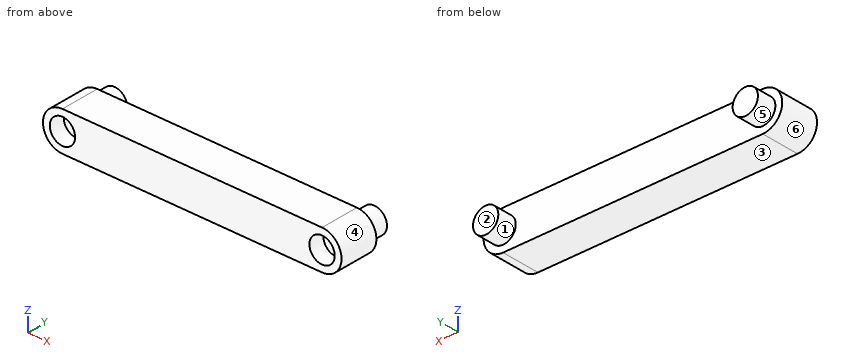
from build123d import *

# Parameters (mm, degrees)
BOSS_EXTRUDE1_DEPTH = 15
SKETCH2_R           = 9.75
CUT_EXTRUDE1_DEPTH  = 117.940155635
BOSS_EXTRUDE2_START = 30
SKETCH2_2_R         = 9.75
BOSS_EXTRUDE2_DEPTH = 30
SKETCH2_3_R         = 9.75
BOSS_EXTRUDE3_DEPTH = 3


with BuildPart() as part:
    # Sketch1 → Boss-Extrude1 (new, symmetric)
    with BuildSketch(Plane(origin=(0, 0, 0), x_dir=(1, 0, 0), z_dir=(0, 1, 0))):
        with BuildLine():
            Line((-100, 15), (100, 15))
            ThreePointArc((100, 15), (115, 0), (100, -15))
            Line((100, -15), (-100, -15))
            ThreePointArc((-100, -15), (-115, 0), (-100, 15))
        make_face()
    extrude(amount=BOSS_EXTRUDE1_DEPTH, both=True)

    # Sketch2 → Cut-Extrude1 (cut, through all)
    with BuildSketch(Plane(origin=(0, 0, 0), x_dir=(1, 0, 0), z_dir=(0, 1, 0))):
        with Locations(Location((100, 0, 0), (0, 0, 270))):
            Circle(SKETCH2_R)
        with Locations(Location((-100, 0, 0), (0, 0, 270))):
            Circle(SKETCH2_R)
    extrude(amount=-CUT_EXTRUDE1_DEPTH, mode=Mode.SUBTRACT)

    # Sketch2_2 → Boss-Extrude2 (add)
    with BuildSketch(Plane(origin=(0, 0, 0), x_dir=(1, 0, 0), z_dir=(0, 1, 0)).offset(BOSS_EXTRUDE2_START)):
        with Locations(Location((100, 0, 0), (0, 0, 270))):
            Circle(SKETCH2_2_R)
        with Locations(Location((-100, 0, 0), (0, 0, 270))):
            Circle(SKETCH2_2_R)
    extrude(amount=-BOSS_EXTRUDE2_DEPTH)

    # Sketch2_3 → Boss-Extrude3 (add)
    with BuildSketch(Plane(origin=(0, 0, 0), x_dir=(1, 0, 0), z_dir=(0, 1, 0))):
        with Locations(Location((100, 0, 0), (0, 0, 270))):
            Circle(SKETCH2_3_R)
        with Locations(Location((-100, 0, 0), (0, 0, 270))):
            Circle(SKETCH2_3_R)
    extrude(amount=-BOSS_EXTRUDE3_DEPTH)


solid = part.part
The model under review builds one solid part; all positions refer to its coordinate system, in mm. Face numbers are marked on the shaded views. A direction names the side the tool comes from. Coordinates: 2 decimals unless noted, no trailing zeros. Write each loop counter-clockwise with the first axis right and the second up, starting at its lowest first coordinate (ties: lowest second). Pieces come first, ordered by that corner, then holes. Notation, with made-up numbers: M 63.5,70 L 121.5,70 A22 ccw 121.5,93 Z; hole C -9,85 d5. An arc over 180 degrees is marked long. Put each result on its own line as item: value.
1) Add section C-C on x = 67. Give the boundary of the cut face in (y, z).
Computed:
outline: M -15,-15 L 15,-15 L 15,15 L -15,15 Z
2) Add section A-A on z = 0. Give the boundary of the cut face in (x, y), then the cut area to 3 significant figures.
Computed:
outline: M -115,-15 L -109.75,-15 L -109.75,-3 L -90.25,-3 L -90.25,-15 L 90.25,-15 L 90.25,-3 L 109.75,-3 L 109.75,-15 L 115,-15 L 115,15 L 109.75,15 L 109.75,30 L 90.25,30 L 90.25,15 L -90.25,15 L -90.25,30 L -109.75,30 L -109.75,15 L -115,15 Z
area: 7,020 mm2
3) Clearance check with flat-ended pins moving along their axes: pin 1 Ø15 at (x, z) = (12.5, 4) entering from +Y; pin 2 Ø3 at (y, z) = (11.5, -5) entering from -X; pin 3 Ø6 at (x, z) = (104.5, 0) entering from -Y; pin 4 Ø12 at (x, y) = (6.5, 24.5) entering from +Z. State where each tip first meets the part, or that it passes through.
Computed:
pin 1: stops at y = 15
pin 2: stops at x = -114.59
pin 3: stops at y = -3
pin 4: passes through
4) Wall thickness on probe 1 along X at (y, z) = (-11.75, 0); probe 2 along Y at (x, z) = (-66, 8.5); probe 3 along X at (y, z) = (-7, -8.5): over which ranges is each line inside the solid? List them lowest first. Write a range as [from, to].
Computed:
probe 1: x = [-115, -109.75], [-90.25, 90.25], [109.75, 115]
probe 2: y = [-15, 15]
probe 3: x = [-112.36, -104.78], [-95.22, 95.22], [104.78, 112.36]
5) Add section B-B on y = 9. Give the boundary of the cut face in (x, z), then the cut area to 3 significant figures.
Computed:
outline: M -100,-15 L 100,-15 A15 ccw 100,15 L -100,15 A15 ccw Z
area: 6,710 mm2
6) Draft analysis for pull direction X (two halves, no side actions). For the marked faces 3, 4, 5 and 6, state which applies: released by +X, released by -X, zero draft, split by the parting line, or undercut.
Computed:
face 3: zero draft
face 4: released by +X
face 5: undercut
face 6: released by -X
7) For the marked faces 1 and 2, list the 3-axis set-ups (+Z, -Z, +X, -X, +Y, -Y) from which the entire face can be reached by the end or side of a thin tool; tool diameter is ignored.
Computed:
face 1: +Y
face 2: +Z, -Z, +X, -X, +Y
